Could you check a few things on this model? Use its own coordinates, in mm. Coordinates: 2 decimals unless noted, no trailing zeros. Order: outer loops, then holes, each group sorted by start corner. A loop starts at its lowest first (then second) coordinate and runs counter-clockwise, first axis right, second up. Notation, with made-up numbers: (48.25, -35.75) - (71.25, -35.75) arc R31 ccw to (71.25, -1.75) - close; hole circle Ø10 at (88.5, 89.25). An arc over 180 degrees is marked (long way). Answer as a JSON object with one key per item and string values. Group by question number.
(1) Please list where these lines run through material, in increasing order: probe 1 along X at (y, z) = (-0.5, -362); probe 2 along X at (y, z) = (-4.25, -383.5); probe 3 along Z at (x, y) = (-177, -0.75).
(2) Will these pins go through, and if not, where does the flat tip stop? P1, Ø1, axis at x = -203, y = -8.5, coming from the +Z side; P2, Ø6, axis at y = -2, z = -574.5, coming from the -X side; P3, Ø5, axis at y = -6, z = -744.5, coming from the -X side.
(3) Imagine slicing it at C-C, the plane x = -393.5. Write out the boundary of the cut face in (y, z).
(4) We'd pull the mould along X, two halves only. Please class faces 1 (the cylindrical face through (-135.65, -4.93, 12.76)), 2 (the flat face through (-316.37, -4.93, -206.51)), 3 (the flat face through (-296.858, -4.93, -601.451)): pulls with the +X half, pulls with the -X half, needs draft (parallel to the pull), parting line crosses it, or undercut.
(5) Imagine slicing it at B-B, the plane z = -734.5. Write out the boundary of the cut face in (x, y), and give its area (3 significant figures).
(6) Imagine slicing it at A-A, the plane y = -5.25. Write out the boundary of the cut face in (x, z).
from build123d import *

# Parameters (mm, degrees)
F0_W     = 100
F0_H     = 100
F0_R     = 15
F1_DEPTH = 10


# Not quite as in the source:
# - a feature names something its author has since deleted; it is built from what else it names


with BuildPart() as f1:
    # F0 (on Front) → F1 (new body)
    with BuildSketch(Plane.XZ):
        with Locations((-366.5186442992, -742.7781961888)):
            Rectangle(F0_W, F0_H)
        with BuildLine():
            Line((-424.891556994, -494.917224318), (-416.5186442992, -692.7781961888))
            Line((-416.5186442992, -692.7781961888), (-316.5186442992, -692.7781961888))
            Line((-316.5186442992, -692.7781961888), (-276.6384194866, -507.5307060219))
            ThreePointArc((-276.6384194866, -507.5307060219), (-356.3167020216, -566.4762885136), (-424.891556994, -494.917224318))
        make_face()
        with BuildLine():
            ThreePointArc((-415.8601836979, -455.9414735734), (-423.022745475, -474.8160209943), (-424.891556994, -494.917224318))
            ThreePointArc((-424.891556994, -494.917224318), (-356.3167020216, -566.4762885136), (-276.6384194866, -507.5307060219))
            ThreePointArc((-276.6384194866, -507.5307060219), (-275.3797520239, -499.6830567418), (-274.9586197372, -491.7462758703))
            ThreePointArc((-274.9586197372, -491.7462758703), (-331.4872540196, -419.0564646962), (-415.8601836979, -455.9414735734))
        make_face()
        with Locations((-349.9586197372, -491.7462758703)):
            Circle(F0_R, mode=Mode.SUBTRACT)
        with BuildLine():
            ThreePointArc((-274.9586197372, -491.7462758703), (-275.3797520239, -499.6830567418), (-276.6384194866, -507.5307060219))
            Line((-276.6384194866, -507.5307060219), (-80.3792470285, -19.7411127776))
            ThreePointArc((-80.3792470285, -19.7411127776), (-177.8494040627, -61.3674231584), (-219.6213859991, 36.0403935367))
            Line((-219.6213859991, 36.0403935367), (-415.8601836979, -455.9414735734))
            ThreePointArc((-415.8601836979, -455.9414735734), (-331.4872540196, -419.0564646962), (-274.9586197372, -491.7462758703))
        make_face()
        with BuildLine():
            ThreePointArc((-219.6213859991, 36.0403935367), (-177.8494040627, -61.3674231584), (-80.3792470285, -19.7411127776))
            ThreePointArc((-80.3792470285, -19.7411127776), (-76.3262459022, -6.0036782783), (-74.9586197372, 8.2537241297))
            ThreePointArc((-74.9586197372, 8.2537241297), (-135.8113138036, 81.9073305236), (-219.6213859991, 36.0403935367))
        make_face()
        with Locations((-149.9586197372, 8.2537241297)):
            Circle(F0_R, mode=Mode.SUBTRACT)
    extrude(amount=F1_DEPTH)


solid = f1.part
Result set:
{
 "1": {"probe 1": "x = -378.39 to -218.09", "probe 2": "x = -386.97 to -226.74", "probe 3": "z = -259.89 to 78.21"},
 "2": {"P1": "stops at z = 61.77", "P2": "stops at x = -421.65", "P3": "stops at x = -416.52"},
 "3": {"outline": "(-10, -792.78) - (0, -792.78) - (0, -399.88) - (-10, -399.88) - close"},
 "4": {"face 1": "undercut", "face 2": "pulls with the -X half", "face 3": "pulls with the +X half"},
 "5": {"outline": "(-416.52, -10) - (-316.52, -10) - (-316.52, 0) - (-416.52, 0) - close", "area": "1,000 mm^2"},
 "6": {"outline": "(-424.89, -494.92) - (-416.52, -692.78) - (-416.52, -792.78) - (-316.52, -792.78) - (-316.52, -692.78) - (-276.64, -507.53) - (-80.38, -19.74) arc R75 ccw to (-219.62, 36.04) - (-415.86, -455.94) arc R75 ccw to start; hole circle Ø30 at (-349.96, -491.75); hole circle Ø30 at (-149.96, 8.25)"}
}
